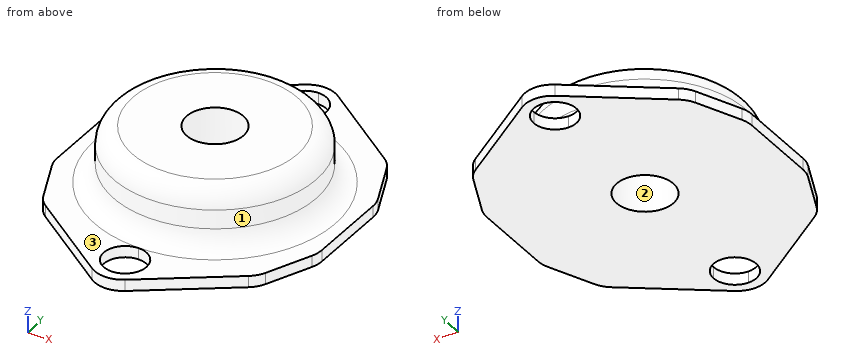
from build123d import *
from build123d.topology import SkipClean

# Parameters (mm, degrees)
EXTRUDE_1_DEPTH     = 1.2
FILLET_1_R          = 3
SKETCH_2_R          = 10.7
EXTRUDE_2_DEPTH     = 6
SKETCH_1_3_R        = 3
CUT_EXTRUDE_1_DEPTH = 20
FILLET_2_R          = 2


with BuildPart() as part:
    # Sketch 1 → Extrude 1 (new body)
    with BuildSketch(Plane.XY):
        with BuildLine():
            Line((-11.411313878, -10.847751594), (0, -19))
            Line((0, -19), (0, -17.25))
            ThreePointArc((0, -17.25), (-2.25, -15), (0, -12.75))
            Line((0, -12.75), (0, -3))
            ThreePointArc((0, -3), (-2.121320344, -2.121320344), (-3, 0))
            ThreePointArc((-3, 0), (-2.121320344, 2.121320344), (0, 3))
            Line((0, 3), (0, 12.75))
            ThreePointArc((0, 12.75), (-2.25, 15), (0, 17.25))
            Line((0, 17.25), (0, 19))
            Line((0, 19), (-11.411313878, 10.847751594))
            Line((-11.411313878, 10.847751594), (-14, 4.917243675))
            Line((-14, 4.917243675), (-14, -4.917243675))
            Line((-14, -4.917243675), (-11.411313878, -10.847751594))
        make_face()
        with BuildLine():
            Line((0, -17.25), (0, -19))
            Line((0, -19), (11.411313878, -10.847751594))
            Line((11.411313878, -10.847751594), (14, -4.917243675))
            Line((14, -4.917243675), (14, 4.917243675))
            Line((14, 4.917243675), (11.411313878, 10.847751594))
            Line((11.411313878, 10.847751594), (0, 19))
            Line((0, 19), (0, 17.25))
            ThreePointArc((0, 17.25), (1.590990258, 16.590990258), (2.25, 15))
            ThreePointArc((2.25, 15), (1.590990258, 13.409009742), (0, 12.75))
            Line((0, 12.75), (0, 3))
            ThreePointArc((0, 3), (2.121320344, 2.121320344), (3, 0))
            ThreePointArc((3, 0), (2.121320344, -2.121320344), (0, -3))
            Line((0, -3), (0, -12.75))
            ThreePointArc((0, -12.75), (1.590990258, -13.409009742), (2.25, -15))
            ThreePointArc((2.25, -15), (1.590990258, -16.590990258), (0, -17.25))
        make_face()
    extrude(amount=EXTRUDE_1_DEPTH)

    # Fillet 1
    fillet_1_edges = [part.edges().sort_by_distance(p)[0] for p in [
        (11.411313878, 10.847751594, 0.6),
        (14, 4.917243675, 0.6),
        (14, -4.917243675, 0.6),
        (11.411313878, -10.847751594, 0.6),
        (0, -19, 0.6),
        (-11.411313878, -10.847751594, 0.6),
        (-14, -4.917243675, 0.6),
        (-14, 4.917243675, 0.6),
        (-11.411313878, 10.847751594, 0.6),
        (0, 19, 0.6),
    ]]
    fillet(fillet_1_edges, radius=FILLET_1_R)

    # Sketch 2 → Extrude 2 (add)
    with BuildSketch(Plane.XY.offset(1.2)):
        Circle(SKETCH_2_R)
    extrude(amount=EXTRUDE_2_DEPTH)

    # Sketch 1_3 → Cut-Extrude 1 (cut)
    with SkipClean():  # the faces are left unmerged after this step: merging them gives an invalid solid
        with BuildSketch(Plane.XY):
            Circle(SKETCH_1_3_R)
        extrude(amount=CUT_EXTRUDE_1_DEPTH, mode=Mode.SUBTRACT)

    # Fillet 2
    fillet_2_edges = [part.edges().sort_by_distance(p)[0] for p in [
        (-10.7, 0, 1.2),
        (-10.7, 0, 7.2),
    ]]
    fillet(fillet_2_edges, radius=FILLET_2_R)


solid = part.part
Verification items for the finished model (mm, model axes). Face numbers are marked on the shaded views. Coordinates: 2 decimals unless noted, no trailing zeros. Order: outer loops, then holes, each group sorted by start corner. A loop starts at its lowest first (then second) coordinate and runs counter-clockwise, first axis right, second up. Notation, with made-up numbers: M 4,65.25 L 40,65.25 A22 ccw 40,73.25 Z; hole C -26,-22 d3. An arc over 180 degrees is marked long. Write each question's results on one line, items separated by ' | '.
1) Scan lines: line 1 along Z through (x, y) = (8.5, 2.5); line 2 along Z through (x, y) = (3.5, -12); line 3 along Y through (x, z) = (1.5, 1.75). Record each from-to range of solid material in increasing order. Write a range as [from, to].
Solved:
line 1: z = [0, 7.19] | line 2: z = [0, 1.21] | line 3: y = [-11.22, -2.6], [2.6, 11.22]
2) Section check C-C on z = 2.25. Record the cut outline in (x, y).
Solved:
outline: C 0,0 d21.88; hole C 0,0 d6
3) Section check B-B on z = 4.75. Record the cut outline in (x, y), plus the area to 3 significant figures.
Solved:
outline: C 0,0 d21.4; hole C 0,0 d6 | area: 331 mm²
4) Gauge pin test, flat ends, axial feed: pin 1 Ø2 at (x, z) = (-2.5, 6.5) entering from -Y; pin 2 Ø3.5 at (x, y) = (0, 0) entering from -Z; pin 3 Ø4 at (x, y) = (-8, -13) entering from +Z; pin 4 Ø1 at (x, y) = (8.5, 10) entering from -Z. Record the tip position at first contact, or that the pin passes through.
Solved:
pin 1: stops at y = -10.47 | pin 2: passes through | pin 3: stops at z = 1.2 | pin 4: stops at z = 0
5) Section check A-A on y = 0. Record the cut outline in (x, z), plus the area to 3 significant figures.
Solved:
outline: M -14,0 L -3,0 L -3,7.2 L -8.7,7.2 A2 ccw -10.7,5.2 L -10.7,3.2 A2 cw -12.7,1.2 L -14,1.2 Z; M 3,0 L 14,0 L 14,1.2 L 12.7,1.2 A2 cw 10.7,3.2 L 10.7,5.2 A2 ccw 8.7,7.2 L 3,7.2 Z | area: 119 mm²
6) Release check for a two-part mould opening along X. For the marked faces 1, 2 and 3 record: pulls with the +X half, pulls with the -X half, needs draft (parallel to the pull), parting line crosses it, or undercut.
Solved:
face 1: parting line crosses it | face 2: undercut | face 3: needs draft
